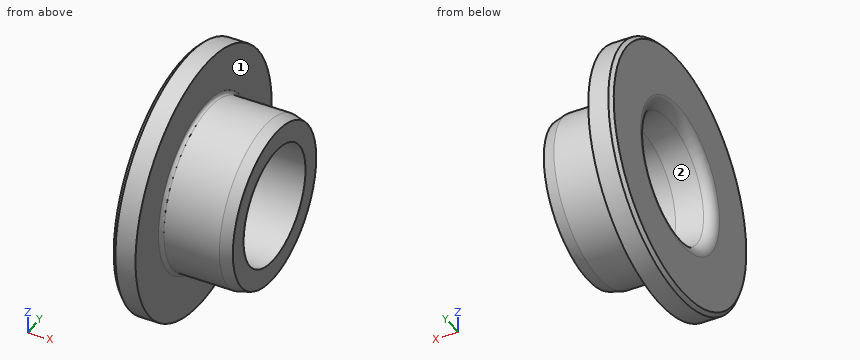
from build123d import *

# Parameters (mm, degrees)
CHAMFER1_SIZE = 0.3
FILLET1_R     = 0.3
FILLET2_R     = 1


with BuildPart() as part:
    # Sketch1 → Revolve1 (revolve)
    with BuildSketch(Plane.XY, mode=Mode.PRIVATE) as revolve1_sk:
        Polygon((-2, 5), (6, 5), (6, 7), (0, 7), (0, 11), (-2, 11), align=None)
    revolve(revolve1_sk.sketch.rotate(Axis((-2, 0, 0), (1, 0, 0)), 90), axis=Axis((-2, 0, 0), (1, 0, 0)))

    # Chamfer1
    chamfer1_edges = [part.edges().sort_by_distance(p)[0] for p in [
        (-2, 0, -11),
    ]]
    chamfer(chamfer1_edges, length=CHAMFER1_SIZE)

    # Fillet1
    fillet1_edges = [part.edges().sort_by_distance(p)[0] for p in [
        (0, 0, -7),
    ]]
    fillet(fillet1_edges, radius=FILLET1_R)

    # Chamfer2: read off the stored shape, not the designer's step
    # Chamfer2 outline → Chamfer2 (revolve, cut)
    with BuildSketch(Plane.YX):
        Polygon((5.528980942, -2), (5, 1), (5, -2), align=None)
    revolve(axis=Axis((0, 0, 0), (1, 0, 0)), mode=Mode.SUBTRACT)

    # Chamfer3: read off the stored shape, not the designer's step
    # Chamfer3 outline → Chamfer3 (revolve, cut)
    with BuildSketch(Plane.YX):
        Polygon((7, 6), (6.732050808, 6), (7, 5), align=None)
    revolve(axis=Axis((0, 0, 0), (1, 0, 0)), mode=Mode.SUBTRACT)

    # Fillet2
    fillet2_edges = [part.edges().sort_by_distance(p)[0] for p in [
        (-2, -5.528980942, 0),
    ]]
    fillet(fillet2_edges, radius=FILLET2_R)


solid = part.part
Could you check a few things on this model? Use its own coordinates, in mm. Face numbers are marked on the shaded views. A direction names the side the tool comes from. Give positions to 0.01 mm unless a question says otherwise; leave off trailing zeros. Order: outer loops, then holes, each group sorted by start corner. A loop starts at its lowest first (then second) coordinate and runs counter-clockwise, first axis right, second up. Notation, with made-up numbers: (-38, -5) - (-3, -5) arc R26 cw to (-3, 11) - close; hole circle Ø10 at (8.25, 70). An arc over 180 degrees is marked (long way). One line per question, with ' | ' between items. Start each with the question number.
Item 1: I'm going to push flat-ended pins straight in: pin 1 Ø5 at (y, z) = (5.5, -8.5) entering from +X; pin 2 Ø9 at (y, z) = (0, 0) entering from +X; pin 3 Ø2 at (x, z) = (3, -4.5) entering from -Y; pin 4 Ø4 at (x, y) = (5, -3.5) entering from +Z. Where does each tip first touch, or does it pass through?
Item 2: I want a section at C-C on x = 2.5. Write out the boundary of the cut face in (y, z).
Item 3: I want a section at A-A on y = 0. Write out the boundary of the cut face in (x, z).
Item 4: I need wall thicknesses on probe 1 along Y at (x, z) = (2.8, 0); probe 2 along X at (y, z) = (6.75, -3); probe 3 along Z at (x, y) = (1.75, 4.25). Which ranges of each line are inside material? Lowest first, please. Write a range as [from, to].
Item 5: For the marked faces 1 and 2, which set-ups out of +Z, -Z, +X, -X, +Y, -Y let a thin tool reach every point of the face, with its end or its side?
Verdict:
1) pin 1: x = 0 | pin 2: through | pin 3: y = -6.06 | pin 4: z = 6.84
2) outline: circle Ø14 at (0, 0); hole circle Ø10 at (0, 0)
3) outline: (-2, -10.7) - (-1.7, -11) - (0, -11) - (0, -7.3) arc R0.3 cw to (0.3, -7) - (5, -7) - (6, -6.73) - (6, -5) - (1, -5) - (-1.17, -5.38) arc R1 ccw to (-2, -6.37) - close; (-2, 6.37) arc R1 ccw to (-1.17, 5.38) - (1, 5) - (6, 5) - (6, 6.73) - (5, 7) - (0.3, 7) arc R0.3 cw to (0, 7.3) - (0, 11) - (-1.7, 11) - (-2, 10.7) - close
4) probe 1: [-7, -5], [5, 7] | probe 2: [-2, 0] | probe 3: [-5.56, -2.63], [2.63, 5.56]
5) face 1: +X | face 2: -X
